The model under review builds one solid part; all positions refer to its coordinate system, in mm. A direction names the side the tool comes from. Round coordinates to 2 decimals unless told otherwise and drop trailing zeros. Write each loop counter-clockwise with the first axis right and the second up, starting at its lowest first coordinate (ties: lowest second). Pieces come first, ordered by that corner, then holes.
Item 1: Add section B-B (y = -8). Give the boundary of the cut face in (x, z), plus the area to 3 significant figures.
Item 2: Machinability: for faces 1 (the face through (18.29, 7.63, 2.46)), 2 (the face through (-1.607, 19.754, 2.465)), 3 (the face through (-3.449, -21.728, 2.465)), 4 (the face through (10.325, -16.992, 2.465)), which of the approach directions +Z, -Z, +X, -X, +Y, -Y give a long, thin tool a straight path to every point of the face, cutting with its end or side? Answer none if there is none.
Item 3: To check wall thickness, follow L1, parallel to X at y = 17, z = 1.65; L2, parallel to X at y = 14, z = 0.5; L3, parallel to Y at x = 19.5, z = 1.45. State the ranges of each line that lie inside material, in increasing order.
Item 4: Add section A-A (x = -2). Give the boundary of the cut face in (y, z), plus the area to 3 significant figures.
```python
from build123d import *

# Parameters (mm, degrees)
BOSS_EXTRUDE1_DEPTH = 5


with BuildPart() as part:
    # Sketch1 → Boss-Extrude1 (new body)
    with BuildSketch(Plane.XY):
        with BuildLine():
            ThreePointArc((-21.806333941, 2.912696354), (-19.784848102, 1.620704589), (-17.471189616, 0.986171591))
            ThreePointArc((-17.471189616, 0.986171591), (-17.499, 0), (-17.471189616, -0.986171591))
            ThreePointArc((-17.471189616, -0.986171591), (-19.784848102, -1.620704589), (-21.806333941, -2.912696354))
            ThreePointArc((-21.806333941, -2.912696354), (-21.729143493, -3.441558231), (-21.639128664, -3.968388926))
            ThreePointArc((-21.639128664, -3.968388926), (-19.317333972, -4.572472634), (-16.920832513, -4.460989585))
            ThreePointArc((-16.920832513, -4.460989585), (-16.642537979, -5.407488385), (-16.31134495, -6.336799421))
            ThreePointArc((-16.31134495, -6.336799421), (-18.31568345, -7.655235955), (-19.838983319, -9.50866662))
            ThreePointArc((-19.838983319, -9.50866662), (-19.602143532, -9.987790994), (-19.353734704, -10.461020648))
            ThreePointArc((-19.353734704, -10.461020648), (-16.958904602, -10.318064378), (-14.714146429, -9.471478019))
            ThreePointArc((-14.714146429, -9.471478019), (-14.156988385, -10.28565413), (-13.554832194, -11.067137173))
            ThreePointArc((-13.554832194, -11.067137173), (-15.05365209, -12.940419489), (-15.929654782, -15.173862347))
            ThreePointArc((-15.929654782, -15.173862347), (-15.556349186, -15.556349186), (-15.173862347, -15.929654782))
            ThreePointArc((-15.173862347, -15.929654782), (-12.940419489, -15.05365209), (-11.067137173, -13.554832194))
            ThreePointArc((-11.067137173, -13.554832194), (-10.28565413, -14.156988385), (-9.471478019, -14.714146429))
            ThreePointArc((-9.471478019, -14.714146429), (-10.318064378, -16.958904602), (-10.461020648, -19.353734704))
            ThreePointArc((-10.461020648, -19.353734704), (-9.987790994, -19.602143532), (-9.50866662, -19.838983319))
            ThreePointArc((-9.50866662, -19.838983319), (-7.655235955, -18.31568345), (-6.336799421, -16.31134495))
            ThreePointArc((-6.336799421, -16.31134495), (-5.407488385, -16.642537979), (-4.460989585, -16.920832513))
            ThreePointArc((-4.460989585, -16.920832513), (-4.572472634, -19.317333972), (-3.968388926, -21.639128664))
            ThreePointArc((-3.968388926, -21.639128664), (-3.441558231, -21.729143493), (-2.912696354, -21.806333941))
            ThreePointArc((-2.912696354, -21.806333941), (-1.620704589, -19.784848102), (-0.986171591, -17.471189616))
            ThreePointArc((-0.986171591, -17.471189616), (0, -17.499), (0.986171591, -17.471189616))
            ThreePointArc((0.986171591, -17.471189616), (1.620704589, -19.784848102), (2.912696354, -21.806333941))
            ThreePointArc((2.912696354, -21.806333941), (3.441558231, -21.729143493), (3.968388926, -21.639128664))
            ThreePointArc((3.968388926, -21.639128664), (4.572472634, -19.317333972), (4.460989585, -16.920832513))
            ThreePointArc((4.460989585, -16.920832513), (5.407488385, -16.642537979), (6.336799421, -16.31134495))
            ThreePointArc((6.336799421, -16.31134495), (7.655235955, -18.31568345), (9.50866662, -19.838983319))
            ThreePointArc((9.50866662, -19.838983319), (9.987790994, -19.602143532), (10.461020648, -19.353734704))
            ThreePointArc((10.461020648, -19.353734704), (10.318064378, -16.958904602), (9.471478019, -14.714146429))
            ThreePointArc((9.471478019, -14.714146429), (10.28565413, -14.156988385), (11.067137173, -13.554832194))
            ThreePointArc((11.067137173, -13.554832194), (12.940419489, -15.05365209), (15.173862347, -15.929654782))
            ThreePointArc((15.173862347, -15.929654782), (15.556349186, -15.556349186), (15.929654782, -15.173862347))
            ThreePointArc((15.929654782, -15.173862347), (15.05365209, -12.940419489), (13.554832194, -11.067137173))
            ThreePointArc((13.554832194, -11.067137173), (14.156988385, -10.28565413), (14.714146429, -9.471478019))
            ThreePointArc((14.714146429, -9.471478019), (16.958904602, -10.318064378), (19.353734704, -10.461020648))
            ThreePointArc((19.353734704, -10.461020648), (19.602143532, -9.987790994), (19.838983319, -9.50866662))
            ThreePointArc((19.838983319, -9.50866662), (18.31568345, -7.655235955), (16.31134495, -6.336799421))
            ThreePointArc((16.31134495, -6.336799421), (16.642537979, -5.407488385), (16.920832513, -4.460989585))
            ThreePointArc((16.920832513, -4.460989585), (19.317333972, -4.572472634), (21.639128664, -3.968388926))
            ThreePointArc((21.639128664, -3.968388926), (21.729143493, -3.441558231), (21.806333941, -2.912696354))
            ThreePointArc((21.806333941, -2.912696354), (19.784848102, -1.620704589), (17.471189616, -0.986171591))
            ThreePointArc((17.471189616, -0.986171591), (17.499, 0), (17.471189616, 0.986171591))
            ThreePointArc((17.471189616, 0.986171591), (19.784848102, 1.620704589), (21.806333941, 2.912696354))
            ThreePointArc((21.806333941, 2.912696354), (21.729143493, 3.441558231), (21.639128664, 3.968388926))
            ThreePointArc((21.639128664, 3.968388926), (19.317333972, 4.572472634), (16.920832513, 4.460989585))
            ThreePointArc((16.920832513, 4.460989585), (16.642537979, 5.407488385), (16.31134495, 6.336799421))
            ThreePointArc((16.31134495, 6.336799421), (18.31568345, 7.655235955), (19.838983319, 9.50866662))
            ThreePointArc((19.838983319, 9.50866662), (19.602143532, 9.987790994), (19.353734704, 10.461020648))
            ThreePointArc((19.353734704, 10.461020648), (16.958904602, 10.318064378), (14.714146429, 9.471478019))
            ThreePointArc((14.714146429, 9.471478019), (14.156988385, 10.28565413), (13.554832194, 11.067137173))
            ThreePointArc((13.554832194, 11.067137173), (15.05365209, 12.940419489), (15.929654782, 15.173862347))
            ThreePointArc((15.929654782, 15.173862347), (15.556349186, 15.556349186), (15.173862347, 15.929654782))
            ThreePointArc((15.173862347, 15.929654782), (12.940419489, 15.05365209), (11.067137173, 13.554832194))
            ThreePointArc((11.067137173, 13.554832194), (10.28565413, 14.156988385), (9.471478019, 14.714146429))
            ThreePointArc((9.471478019, 14.714146429), (10.318064378, 16.958904602), (10.461020648, 19.353734704))
            ThreePointArc((10.461020648, 19.353734704), (9.987790994, 19.602143532), (9.50866662, 19.838983319))
            ThreePointArc((9.50866662, 19.838983319), (7.655235955, 18.31568345), (6.336799421, 16.31134495))
            ThreePointArc((6.336799421, 16.31134495), (5.407488385, 16.642537979), (4.460989585, 16.920832513))
            ThreePointArc((4.460989585, 16.920832513), (4.572472634, 19.317333972), (3.968388926, 21.639128664))
            ThreePointArc((3.968388926, 21.639128664), (3.441558231, 21.729143493), (2.912696354, 21.806333941))
            ThreePointArc((2.912696354, 21.806333941), (1.620704589, 19.784848102), (0.986171591, 17.471189616))
            ThreePointArc((0.986171591, 17.471189616), (0, 17.499), (-0.986171591, 17.471189616))
            ThreePointArc((-0.986171591, 17.471189616), (-1.620704589, 19.784848102), (-2.912696354, 21.806333941))
            ThreePointArc((-2.912696354, 21.806333941), (-3.441558231, 21.729143493), (-3.968388926, 21.639128664))
            ThreePointArc((-3.968388926, 21.639128664), (-4.572472634, 19.317333972), (-4.460989585, 16.920832513))
            ThreePointArc((-4.460989585, 16.920832513), (-5.407488385, 16.642537979), (-6.336799421, 16.31134495))
            ThreePointArc((-6.336799421, 16.31134495), (-7.655235955, 18.31568345), (-9.50866662, 19.838983319))
            ThreePointArc((-9.50866662, 19.838983319), (-9.987790994, 19.602143532), (-10.461020648, 19.353734704))
            ThreePointArc((-10.461020648, 19.353734704), (-10.318064378, 16.958904602), (-9.471478019, 14.714146429))
            ThreePointArc((-9.471478019, 14.714146429), (-10.28565413, 14.156988385), (-11.067137173, 13.554832194))
            ThreePointArc((-11.067137173, 13.554832194), (-12.940419489, 15.05365209), (-15.173862347, 15.929654782))
            ThreePointArc((-15.173862347, 15.929654782), (-15.556349186, 15.556349186), (-15.929654782, 15.173862347))
            ThreePointArc((-15.929654782, 15.173862347), (-15.05365209, 12.940419489), (-13.554832194, 11.067137173))
            ThreePointArc((-13.554832194, 11.067137173), (-14.156988385, 10.28565413), (-14.714146429, 9.471478019))
            ThreePointArc((-14.714146429, 9.471478019), (-16.958904602, 10.318064378), (-19.353734704, 10.461020648))
            ThreePointArc((-19.353734704, 10.461020648), (-19.602143532, 9.987790994), (-19.838983319, 9.50866662))
            ThreePointArc((-19.838983319, 9.50866662), (-18.31568345, 7.655235955), (-16.31134495, 6.336799421))
            ThreePointArc((-16.31134495, 6.336799421), (-16.642537979, 5.407488385), (-16.920832513, 4.460989585))
            ThreePointArc((-16.920832513, 4.460989585), (-19.317333972, 4.572472634), (-21.639128664, 3.968388926))
            ThreePointArc((-21.639128664, 3.968388926), (-21.729143493, 3.441558231), (-21.806333941, 2.912696354))
        make_face()
    extrude(amount=BOSS_EXTRUDE1_DEPTH)


solid = part.part
```
Numbers:
1. outline: (-18.68, 0) - (18.68, 0) - (18.68, 5) - (-18.68, 5) - close
1. area: 187 mm2
2. face 1: +Z, -Z, +X
2. face 2: +Z, -Z, +Y
2. face 3: +Z, -Z, -X, -Y
2. face 4: +Z, -Z
3. L1: x = -10.33 to -6.7, -4.48 to 4.48, 6.7 to 10.33
3. L2: x = -15.57 to -11.51, -10.5 to 10.5, 11.51 to 15.57
3. L3: y = -10.19 to -8.99, -4.55 to -1.5, 1.5 to 4.55, 8.99 to 10.19
4. outline: (-20.53, 0) - (20.53, 0) - (20.53, 5) - (-20.53, 5) - close
4. area: 205 mm2
